from build123d import *

# Parameters (mm, degrees)
F0_W          = 57
F0_H          = 27
F0_W_2        = 46
F0_H_2        = 25
F1_DEPTH      = 13
F2_DEPTH      = 2.5
F3_W          = 10
F3_H          = 3
F4_DEPTH      = 46
F5_R          = 1.5
F6_DEPTH      = 5.501
F6_DEPTH_BACK = 51.501
F7_SIZE       = 1.5
F8_R          = 1.5
F9_DEPTH      = 3.5
F10_R         = 3.5
F10_R_2       = 1.5
F11_DEPTH     = 3.7
F13_DEPTH     = 46
F14_R         = 1.2
F15_DEPTH     = 57.001
F16_R         = 0.75
F17_DEPTH     = 6
F18_T1_DEPTH  = 47.5734639037
F19_W         = 1
F19_H         = 4
F19_H_2       = 1.5
F19_W_2       = 1.5
F19_H_3       = 1
F20_DEPTH     = 0.3
F21_R         = 1


# Not quite as in the source:
# - a fillet or chamfer that OpenCascade refuses, or shapes differently, is made with other operations: its cross-section is extruded or revolved along the edge and cut away or added


with BuildPart() as f1:
    # F0 (on Front) → F1 (new body)
    with BuildSketch(Plane.XZ):
        Rectangle(F0_W, F0_H)
        Rectangle(F0_W_2, F0_H_2, mode=Mode.SUBTRACT)
    extrude(amount=F1_DEPTH)

    # F0 (on Front) → F2 (join)
    with BuildSketch(Plane.XZ):
        Rectangle(F0_W_2, F0_H_2)
    extrude(amount=F2_DEPTH)

    # F3 (on face) → F4 (join, through all)
    with BuildSketch(Plane.YZ.offset(-23)):
        with Locations((-6, 0)):
            Rectangle(F3_W, F3_H)
    extrude(amount=F4_DEPTH)

    # F5 (on face) → F6 (cut, two sides)
    with BuildSketch(Plane.YZ.offset(-23)) as f6_sk:
        with Locations((-8.3, 6.6)):
            Circle(F5_R)
        with Locations((-8.3, -6.6)):
            Circle(F5_R)
    extrude(amount=-F6_DEPTH, mode=Mode.SUBTRACT)
    extrude(f6_sk.sketch, amount=F6_DEPTH_BACK, mode=Mode.SUBTRACT)

    # F7
    f7_edges = [f1.edges().sort_by_distance(p)[0] for p in [
        (-23, -9.8, 6.6),
        (-23, -9.8, -6.6),
        (23, -9.8, 6.6),
        (23, -9.8, -6.6),
    ]]
    chamfer(f7_edges, length=F7_SIZE)

    # F8 (on face) → F9 (cut)
    with BuildSketch(Plane(origin=(-28.5, 0, 0), x_dir=(0, -1, 0), z_dir=(-1, 0, 0))):
        Polygon((6.5679491924, -3.6), (4.8358983849, -6.6), (6.5679491924, -9.6), (10.0320508076, -9.6), (11.7641016151, -6.6), (10.0320508076, -3.6), align=None)
        with Locations((8.3, -6.6)):
            Circle(F8_R, mode=Mode.SUBTRACT)
        Polygon((10.0320508076, 9.6), (6.5679491924, 9.6), (4.8358983849, 6.6), (6.5679491924, 3.6), (10.0320508076, 3.6), (11.7641016151, 6.6), align=None)
        with Locations((8.3, 6.6)):
            Circle(F8_R, mode=Mode.SUBTRACT)
        with Locations((8.3, 6.6)):
            Circle(F8_R)
    extrude(amount=-F9_DEPTH, mode=Mode.SUBTRACT)

    # F10 (on face) → F11 (cut)
    with BuildSketch(Plane.YZ.offset(28.5)):
        with Locations((-8.3, 6.6)):
            Circle(F10_R)
        with Locations((-8.3, 6.6)):
            Circle(F10_R_2, mode=Mode.SUBTRACT)
        with Locations((-8.3, -6.6)):
            Circle(F10_R)
        with Locations((-8.3, -6.6)):
            Circle(F10_R_2, mode=Mode.SUBTRACT)
    extrude(amount=-F11_DEPTH, mode=Mode.SUBTRACT)

    # F12 (on face) → F13 (join, through all)
    with BuildSketch(Plane.YZ.offset(-23)):
        with BuildLine():
            Line((-2.5, -12.5), (-2.5, -10.5))
            ThreePointArc((-2.5, -10.5), (-3.3173241863, -11.6826758137), (-4.5, -12.5))
            Line((-4.5, -12.5), (-2.5, -12.5))
        make_face()
        with BuildLine():
            ThreePointArc((-4.5, -1.5), (-3.3173241863, -2.3173241863), (-2.5, -3.5))
            Line((-2.5, -3.5), (-2.5, -1.5))
            Line((-2.5, -1.5), (-4.5, -1.5))
        make_face()
        with BuildLine():
            Line((-2.5, 12.5), (-4.5, 12.5))
            ThreePointArc((-4.5, 12.5), (-3.3173241863, 11.6826758137), (-2.5, 10.5))
            Line((-2.5, 10.5), (-2.5, 12.5))
        make_face()
        with BuildLine():
            ThreePointArc((-2.5, 3.5), (-3.3173241863, 2.3173241863), (-4.5, 1.5))
            Line((-4.5, 1.5), (-2.5, 1.5))
            Line((-2.5, 1.5), (-2.5, 3.5))
        make_face()
    extrude(amount=F13_DEPTH)

    # F14 (on face) → F15 (cut, through all)
    with BuildSketch(Plane.YZ.offset(28.5)):
        with Locations((-1.55, 0)):
            Circle(F14_R)
    extrude(amount=-F15_DEPTH, mode=Mode.SUBTRACT)

    # F16 (on face) → F17 (cut)
    with BuildSketch(Plane(origin=(0, 0, 0), x_dir=(-1, 0, 0), z_dir=(0, 1, 0))):
        with Locations((-25.85, -6.6)):
            Circle(F16_R)
        with Locations((-25.85, 6.6)):
            Circle(F16_R)
        with Locations((25.85, 6.6)):
            Circle(F16_R)
        with Locations((25.85, -6.6)):
            Circle(F16_R)
    extrude(amount=-F17_DEPTH, mode=Mode.SUBTRACT)

    # F18: chamfer of 4 on 2 edges, made by hand

    # F18_s2 → F18_t1 (cut)
    with BuildSketch(Plane.XY.offset(-23.7867319519)):
        Polygon((24.5, 0), (28.5, -4), (28.5, 0), align=None)
        Polygon((-28.5, -4), (-24.5, 0), (-28.5, 0), align=None)
    extrude(amount=F18_T1_DEPTH, mode=Mode.SUBTRACT)

    # F19 (on face) → F20 (cut)
    with BuildSketch(Plane.XZ.offset(13)):
        with Locations((25.75, -6.6)):
            Rectangle(F19_W, F19_H)
        with Locations((25.75, 6.6)):
            Rectangle(F19_W, F19_H)
        with Locations((-25.75, 5.35)):
            Rectangle(F19_W, F19_H_2)
        with Locations((-27, 6.6)):
            Rectangle(F19_W_2, F19_H_3)
        with Locations((-25.75, 6.6)):
            Rectangle(F19_W, F19_H_3)
        with Locations((-24.5, 6.6)):
            Rectangle(F19_W_2, F19_H_3)
        with Locations((-25.75, 7.85)):
            Rectangle(F19_W, F19_H_2)
        with Locations((-25.75, -5.35)):
            Rectangle(F19_W, F19_H_2)
        with Locations((-24.5, -6.6)):
            Rectangle(F19_W_2, F19_H_3)
        with Locations((-25.75, -6.6)):
            Rectangle(F19_W, F19_H_3)
        with Locations((-27, -6.6)):
            Rectangle(F19_W_2, F19_H_3)
        with Locations((-25.75, -7.85)):
            Rectangle(F19_W, F19_H_2)
    extrude(amount=-F20_DEPTH, mode=Mode.SUBTRACT)

    # F21
    f21_edges = [f1.edges().sort_by_distance(p)[0] for p in [
        (0, -11, -1.5),
        (0, -11, 1.5),
    ]]
    fillet(f21_edges, radius=F21_R)


solid = f1.part
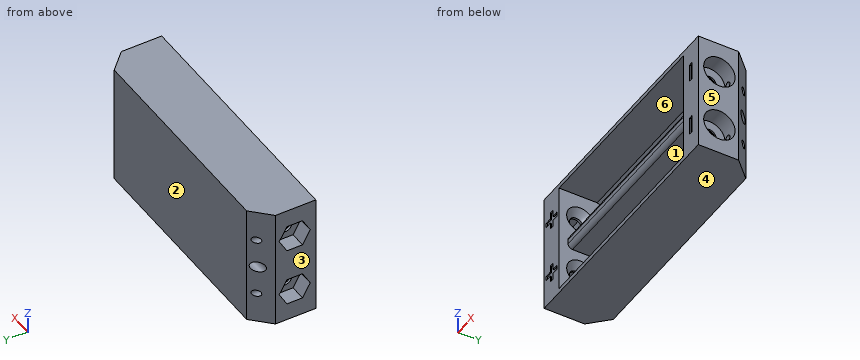
Could you check a few things on this model? Use its own coordinates, in mm. Face numbers are marked on the shaded views. A direction names the side the tool comes from. Coordinates: 2 decimals unless noted, no trailing zeros. Write each loop counter-clockwise with the first axis right and the second up, starting at its lowest first coordinate (ties: lowest second). Pieces come first, ordered by that corner, then holes. Notation, with made-up numbers: (28, 49) - (44, 49) arc R29 cw to (44, 72) - close; hole circle Ø1 at (4, -33). An arc over 180 degrees is marked (long way). Write item = value, one per line.
1) Suppose I cut it at C-C on y = -8.3. State how many separate pieces and enclosed holes the cut face has, plus the area to 3 significant figures.
Result set:
separate_pieces = 3
enclosed_holes = 0
area = 401 mm2
2) Suppose I cut it at B-B on y = -1.55. Please give me the cut outline in (x, z).
Result set:
outline = (-26.05, -13.5) - (26.05, -13.5) - (26.05, -7.32) arc R0.75 cw (long way) to (26.05, -5.88) - (26.05, -1.2) - (-26.05, -1.2) - (-26.05, -5.88) arc R0.75 cw (long way) to (-26.05, -7.32) - close; (-26.05, 1.2) - (26.05, 1.2) - (26.05, 5.88) arc R0.75 cw (long way) to (26.05, 7.32) - (26.05, 13.5) - (-26.05, 13.5) - (-26.05, 7.32) arc R0.75 cw (long way) to (-26.05, 5.88) - close
3) Will these pins go through, and if not, where does the flat tip stop? pin 1 Ø1 at (y, z) = (-2, 3) entering from -X; pin 2 Ø3.5 at (y, z) = (-7.5, -7.5) entering from +X.
Result set:
pin_1 = -27
pin_2 = 24.8
4) For the marked faces 1 and 2, which set-ups out of +Z, -Z, +X, -X, +Y, -Y let a thin tool reach every point of the face, with its end or its side?
Result set:
face_1 = -Y
face_2 = +Z, -Z, +X, -X, +Y
5) We'd pull the mould along X, two halves only. Please class the marked faces 3, 4, 5 and 6: +X half, -X half, draft (parallel to the pull), parting line (faces both ways), or undercut.
Result set:
face_3 = -X half
face_4 = draft
face_5 = +X half
face_6 = undercut
6) Please list where these lines run through material, in increasing order: line 1 (Z direction, x = -24.8, y = -8.3); line 2 (Z direction, x = 1, y = -5.5); line 3 (X direction, y = -4, z = -11.5). Write a range as [from, to].
Result set:
line_1 = [-13.5, -8.1], [-5.1, 5.1], [8.1, 13.5]
line_2 = [-13.5, -12.5], [-1.5, 1.5], [12.5, 13.5]
line_3 = [-28.5, -23], [23, 28.5]
7) Suppose I cut it at A-A on x = 18.5. Please give me the cut outline in (y, z).
Result set:
outline = (-13, -13.5) - (0, -13.5) - (0, 13.5) - (-13, 13.5) - (-13, 12.5) - (-4.5, 12.5) arc R4 cw to (-2.5, 10.5) - (-2.5, 3.5) arc R4 cw to (-4.5, 1.5) - (-10, 1.5) arc R1 ccw to (-11, 0.5) - (-11, -0.5) arc R1 ccw to (-10, -1.5) - (-4.5, -1.5) arc R4 cw to (-2.5, -3.5) - (-2.5, -10.5) arc R4 cw to (-4.5, -12.5) - (-13, -12.5) - close; hole circle Ø2.4 at (-1.55, 0)
